CAD build for the part. Positions are in the model's coordinates, mm. A direction names the side the tool comes from. Round coordinates to 2 decimals unless told otherwise and drop trailing zeros. Loops run counter-clockwise (first coordinate to the right, second up) from the corner with the lowest first, then second, coordinate; pieces in that order, holes last.
```python
from build123d import *

# Parameters (mm, degrees)
BOSS_EXTRUDE1_DEPTH = 5
BOSS_EXTRUDE2_START = 5
SKETCH2_2_W         = 40
SKETCH2_2_H         = 9
BOSS_EXTRUDE2_DEPTH = 1
CUT_EXTRUDE1_REACH  = 25.265
SKETCH3_R           = 3.175
SKETCH7_R           = 2.5
SKETCH7_R_2         = 1.5
CUT_EXTRUDE2_DEPTH  = 2
SKETCH7_3_R         = 1.5
CUT_EXTRUDE3_DEPTH  = 23.737634002
CHAMFER1_SIZE       = 1


with BuildPart() as part:
    # Sketch2 → Boss-Extrude1 (new, symmetric)
    with BuildSketch(Plane.XY):
        Polygon((-10, 4.5), (10, 4.5), (20, 4.5), (20, -4.5), (10, -4.5), (-10, -4.5), (-20, -4.5), (-20, 4.5), align=None)
        with BuildLine():
            Line((-10, 3.5), (10, 3.5))
            ThreePointArc((10, 3.5), (13.5, 0), (10, -3.5))
            Line((10, -3.5), (-10, -3.5))
            ThreePointArc((-10, -3.5), (-13.5, 0), (-10, 3.5))
        make_face(mode=Mode.SUBTRACT)
    extrude(amount=BOSS_EXTRUDE1_DEPTH, both=True)

    # Sketch2_2 → Boss-Extrude2 (add)
    with BuildSketch(Plane.XY.offset(BOSS_EXTRUDE2_START)):
        Rectangle(SKETCH2_2_W, SKETCH2_2_H)
    extrude(amount=BOSS_EXTRUDE2_DEPTH)

    # Sketch3 → Cut-Extrude1 (cut, up to next)
    with BuildSketch(Plane.XY.offset(6), mode=Mode.PRIVATE) as cut_extrude1_sk1:
        Circle(SKETCH3_R)
    cut_extrude1_tool1 = extrude(cut_extrude1_sk1.sketch, amount=-CUT_EXTRUDE1_REACH, mode=Mode.PRIVATE) & part.part
    add(cut_extrude1_tool1.solids().sort_by_distance((0, 0, 6))[0], mode=Mode.SUBTRACT)

    # Sketch7 → Cut-Extrude2 (cut)
    # profile 1 of 4: a face of its own
    with BuildSketch(Plane(origin=(0, 4.5, 0), x_dir=(1, 0, 0), z_dir=(0, 1, 0))):
        with Locations(Location((16, 0, 0), (0, 0, 270))):
            Circle(SKETCH7_R)
    # profile 2 of 4: a face of its own
    with BuildSketch(Plane(origin=(0, 4.5, 0), x_dir=(1, 0, 0), z_dir=(0, 1, 0))):
        with Locations((16, 0)):
            Circle(SKETCH7_R_2)
    # profile 3 of 4: a face of its own
    with BuildSketch(Plane(origin=(0, 4.5, 0), x_dir=(1, 0, 0), z_dir=(0, 1, 0))):
        with Locations(Location((-16, 0, 0), (0, 0, 270))):
            Circle(SKETCH7_R)
        with Locations((-16, 0)):
            Circle(SKETCH7_R_2, mode=Mode.SUBTRACT)
    # profile 4 of 4: a face of its own
    with BuildSketch(Plane(origin=(0, 4.5, 0), x_dir=(1, 0, 0), z_dir=(0, 1, 0))):
        with Locations((-16, 0)):
            Circle(SKETCH7_R_2)
    extrude(amount=-CUT_EXTRUDE2_DEPTH, mode=Mode.SUBTRACT)

    # Sketch7_3 → Cut-Extrude3 (cut, through all)
    with BuildSketch(Plane(origin=(0, 4.5, 0), x_dir=(1, 0, 0), z_dir=(0, 1, 0))):
        with Locations(Location((-16, 0, 0), (0, 0, 270))):
            Circle(SKETCH7_3_R)
        with Locations(Location((16, 0, 0), (0, 0, 270))):
            Circle(SKETCH7_3_R)
    extrude(amount=-CUT_EXTRUDE3_DEPTH, mode=Mode.SUBTRACT)

    # Chamfer1
    chamfer1_edges = [part.edges().sort_by_distance(p)[0] for p in [
        (20, 4.5, 0.5),
        (20, -4.5, 0.5),
        (-20, -4.5, 0.5),
        (-20, 4.5, 0.5),
    ]]
    chamfer(chamfer1_edges, length=CHAMFER1_SIZE)


solid = part.part
```
Item 1: Cut at C-C, the plane x = 16. Give the cut face in (y, z).
Answers follow:
outline: (-4.5, -5) - (4.5, -5) - (4.5, -2.5) - (2.5, -2.5) - (2.5, -1.5) - (-4.5, -1.5) - close; (-4.5, 1.5) - (2.5, 1.5) - (2.5, 2.5) - (4.5, 2.5) - (4.5, 6) - (-4.5, 6) - close
Item 2: Cut at D-D, the plane z = -4. Give the cut face in (x, y).
Answers follow:
outline: (-20, -3.5) - (-19, -4.5) - (19, -4.5) - (20, -3.5) - (20, 3.5) - (19, 4.5) - (-19, 4.5) - (-20, 3.5) - close; hole (-10, -3.5) - (10, -3.5) arc R3.5 ccw to (10, 3.5) - (-10, 3.5) arc R3.5 ccw to start
Item 3: Cut at A-A, the plane z = 0. Give the cut face in (x, y), plus the area to 3 significant figures.
Answers follow:
outline: (-20, -3.5) - (-19, -4.5) - (-17.5, -4.5) - (-17.5, 2.5) - (-18.5, 2.5) - (-18.5, 4.5) - (-19, 4.5) - (-20, 3.5) - close; (-14.5, -4.5) - (14.5, -4.5) - (14.5, 2.5) - (13.5, 2.5) - (13.5, 4.5) - (-13.5, 4.5) - (-13.5, 2.5) - (-14.5, 2.5) - close; (17.5, -4.5) - (19, -4.5) - (20, -3.5) - (20, 3.5) - (19, 4.5) - (18.5, 4.5) - (18.5, 2.5) - (17.5, 2.5) - close; hole (-10, -3.5) - (10, -3.5) arc R3.5 ccw to (10, 3.5) - (-10, 3.5) arc R3.5 ccw to start
area: 118 mm2
Item 4: Flat gauge pins, fed straight in: P1, Ø4, axis at x = -16, z = 0, coming from the +Y side; P2, Ø2, axis at x = -3.5, y = 1, coming from the -Z side. Where does each tip first touch, or does it go through?
Answers follow:
P1: stops at y = 2.5
P2: stops at z = 5
Item 5: Probe line 1 (Y direction, x = 2.5, z = 2.75); line 2 (X direction, y = 4, z = 0); line 3 (X direction, y = 3.2, z = 0). List the from-to ranges inside material, lowest first.
Answers follow:
line 1: y = -4.5 to -3.5, 3.5 to 4.5
line 2: x = -19.5 to -18.5, -13.5 to 13.5, 18.5 to 19.5
line 3: x = -20 to -18.5, -13.5 to -11.42, 11.42 to 13.5, 18.5 to 20
Item 6: 3-axis set-ups, long thin cutter, end or side, ignore diameter. For faces 4 (the cylindrical face through (-15.55, -0.95, 1.43)), 5 (the cylindrical face through (-13.5, -0.1, 0.1)), 6 (the cylindrical face through (13.78, 3.51, 1.15)): which of +Z, -Z, +X, -X, +Y, -Y reach the whole face in a straight line?
Answers follow:
face 4: +Y, -Y
face 5: -Z
face 6: +Y
Item 7: Cut at B-B, the plane y = 0. Give the cut face in (x, z) (3 decimals), plus the area to 3 significant figures.
Answers follow:
outline: (-20, -5) - (-13.5, -5) - (-13.5, 5) - (-3.175, 5) - (-3.175, 6) - (-20, 6) - close; (3.175, 5) - (13.5, 5) - (13.5, -5) - (20, -5) - (20, 6) - (3.175, 6) - close; hole circle Ø3 at (-16, 0); hole circle Ø3 at (16, 0)
area: 150 mm2
Item 8: Two-plate mould, pull along Y, no slides. Class faces 1 (the cylindrical face through (-0.69, -3.1, 5.51)), 2 (the cylindrical face through (17.265, -0.951, 0.806)), 3 (the flat face through (19.5, -4, 0.4)): released by +Y, released by -Y, zero draft, split by the parting line, or undercut.
Answers follow:
face 1: undercut
face 2: zero draft
face 3: released by -Y
